Autodesk Inventor part; units mm, degrees
ref_plane "РабПлоскость1" through (0, 1.5, 0) normal (0, -1, 0) x (1, 0, 0)
ref_plane "YZ Plane" through (0, 0, 0) normal (1, 0, 0) x (0, 1, 0)
ref_plane "XZ Plane" through (0, 0, 0) normal (0, 1, 0) x (-1, 0, 0)
sketch "Эскиз1" plane through (0, 0, 0) normal (0, 1, 0) x (-1, 0, 0)
  circle A0 centre (0, 0) radius 8
  circle A1 centre (0, 0) radius 2.5
  circle A2 centre (0, 0) radius 4
  circle A3 centre (0, 0) radius 6
  dimension "d0" = 16
  dimension "d1" = 5
  dimension "d2" = 8
  dimension "d3" = 12
extrude "Выдавливание1" add sketch "Эскиз1" along normal blind 5
chamfer "Фаска1" distance 0.25 angle 45 8 edges at (8, 0, 0) (8, 5, 0) (6, 5, 0) (2.5, 0, 0) (2.5, 5, 0) (4, 5, 0) (4, 0, 0) (6, 0, 0)
ref_plane "РабПлоскость1" through (0, 1.5, 0) normal (0, -1, 0) x (1, 0, 0)
sketch "Эскиз2" plane through (0, 1.5, 0) normal (0, -1, 0) x (1, 0, 0)
  circle A0 centre (0, 0) radius 6.25
  circle A1 centre (0, 0) radius 6.7619
  circle A2 centre (0, 0) radius 3.4801
extrude "Выдавливание2" add sketch "Эскиз2" against normal blind 2 contours A0
properties part number "625zz"
The listing builds one solid part. Answer for the finished solid, in the listing's coordinates (mm). A direction names the side the tool comes from. Round coordinates to 2 decimals unless told otherwise and drop trailing zeros. Write each loop counter-clockwise with the first axis right and the second up, starting at its lowest first coordinate (ties: lowest second). Pieces come first, ordered by that corner, then holes. Notation, with made-up numbers: (30.25, 86) -> (39.25, 86) arc R29 cw to (39.25, 122) -> close; hole circle Ø3 at (-28, 1.5). An arc over 180 degrees is marked (long way). Write item = value, one per line.
1) Section B-B on y = 2.6 is taken. Write down the section's boundary in (x, z).
Check values:
outline = circle Ø16 at (0, 0); hole circle Ø5 at (0, 0)
2) Straight lines are drawn through the part: line 1 along Z through (x, y) = (0, 1.2); line 2 along Z through (x, y) = (-2.25, 1.2); line 3 along Z through (x, y) = (2.75, 1.4). For each, find the intervals that lie inside material, in ascending order. Write a range as [from, to].
Check values:
line_1 = [-8, -6], [-4, -2.5], [2.5, 4], [6, 8]
line_2 = [-7.68, -5.56], [-3.31, -1.09], [1.09, 3.31], [5.56, 7.68]
line_3 = [-7.51, -5.33], [-2.9, 2.9], [5.33, 7.51]
3) For a pull along Z with two mould halves and no side action, classify faces 4 (the cylindrical face through (6, 4, 0)), 5 (the cylindrical face through (1.73, 2.47, 7.81)), 6 (the flat face through (1, 0, 3)) as released by +Z, released by -Z, zero draft, split by the parting line, or undercut.
Check values:
face_4 = undercut
face_5 = split by the parting line
face_6 = zero draft
4) Section A-A on y = 4.55 is taken. Write down the section's boundary in (x, z).
Check values:
outline = circle Ø16 at (0, 0); circle Ø8 at (0, 0); hole circle Ø12 at (0, 0); hole circle Ø5 at (0, 0)
5) Given pin 1 (6 mm diameter, centred on x = -2.5, z = 0.5, fed in from -Y); pin 2 (3 mm diameter, centred on y = 2.5, z = 3, fed in from -X); pin 3 (3 mm diameter, centred on x = 5.5, y = 3, fed in from -Z); pin 4 (1 mm diameter, centred on x = 0.5, z = 5, fed in from +Y), each flat-ended and moving along its own axis, determine where each tip first touches the part or whether it passes through.
Check values:
pin_1 = 0
pin_2 = -7.86
pin_3 = -6.93
pin_4 = 3.5
6) Which of the six approach directions +Z, -Z, +X, -X, +Y, -Y give full straight-line access (tool end or side, diameter ignored) to faces 1 (the flat face through (-0.5, 5, 6.4)), 2 (the cylindrical face through (6, 1, 0)), 3 (the flat face through (-1.42, 3.5, -3.92))?
Check values:
face_1 = +Z, -Z, +X, -X, +Y
face_2 = -Y
face_3 = +Y
